```python
from build123d import *

# Parameters (mm, degrees)
BASPROSKE_W             = 12
BASPROSKE_H             = 25.5
TOOTHCUT_DEPTH          = 39.006578378
TEETHCUTS_COUNT         = 15
TEETHCUTS_ANGLE         = 336
BORSKE_R                = 10
BORE_DEPTH              = 50.0000508
CUT_EXTRUDE1_DEPTH      = 38.954121274
CUT_EXTRUDE1_DEPTH_BACK = 38.954121274
SKETCH1_W               = 6
SKETCH1_H               = 6


with BuildPart() as part:
    # BasProSke → Base-Revolve (revolve)
    with BuildSketch(Plane(origin=(0, 0, 0), x_dir=(1, 0, 0), z_dir=(0, 1, 0)), mode=Mode.PRIVATE) as base_revolve_sk:
        with Locations((6, 12.75)):
            Rectangle(BASPROSKE_W, BASPROSKE_H)
    revolve(base_revolve_sk.sketch.rotate(Axis((-10, 0, 0), (1, 0, 0)), 180), axis=Axis((-10, 0, 0), (1, 0, 0)))

    # TooCutSke → ToothCut (cut, through all)
    with BuildSketch(Plane(origin=(0, 0, 0), x_dir=(0, 0, -1), z_dir=(1, 0, 0))):
        with BuildLine():
            ThreePointArc((1.584594428, 18.681918036), (0, 18.749), (-1.584594428, 18.681918036))
            ThreePointArc((-1.584594428, 18.681918036), (-2.465052499, 22.206073835), (-4.666912141, 25.095138498))
            ThreePointArc((-4.666912141, 25.095138498), (0, 25.5254), (4.666912141, 25.095138498))
            ThreePointArc((4.666912141, 25.095138498), (2.465052499, 22.206073835), (1.584594428, 18.681918036))
        make_face()
    toothcut = extrude(amount=TOOTHCUT_DEPTH, mode=Mode.SUBTRACT)

    # TeethCuts: ToothCut ×15 about axis
    teethcuts_axis = Axis((-10, 0, 0), (1, 0, 0))
    for i in range(1, TEETHCUTS_COUNT):
        add(toothcut.rotate(teethcuts_axis, i * TEETHCUTS_ANGLE / (TEETHCUTS_COUNT - 1)), mode=Mode.SUBTRACT)

    # BorSke → Bore (cut, symmetric)
    with BuildSketch(Plane(origin=(0, 0, 0), x_dir=(0, 0, -1), z_dir=(1, 0, 0))):
        with Locations(Location((0, 0, 0), (0, 0, 180))):
            Circle(BORSKE_R)
    extrude(amount=BORE_DEPTH, both=True, mode=Mode.SUBTRACT)

    # Sketch1 → Cut-Extrude1 (cut, two sides: drawn at the far end of the back side and taken through both)
    with BuildSketch(Plane(origin=(0, 0, 0), x_dir=(0, 0, -1), z_dir=(1, 0, 0)).offset(-CUT_EXTRUDE1_DEPTH_BACK)):
        with Locations((0, 10)):
            Rectangle(SKETCH1_W, SKETCH1_H)
    extrude(amount=CUT_EXTRUDE1_DEPTH + CUT_EXTRUDE1_DEPTH_BACK, mode=Mode.SUBTRACT)


solid = part.part
```
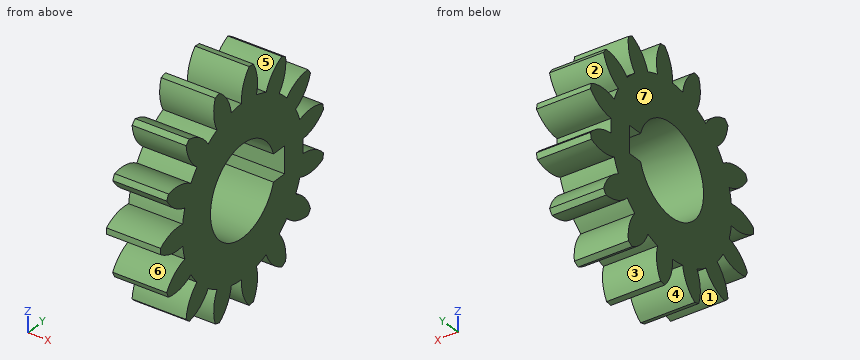
Work out the finished part from the listing and answer in its coordinate system (mm). Face numbers are marked on the shaded views. A direction names the side the tool comes from. Coordinates: 2 decimals unless noted, no trailing zeros. Loops run counter-clockwise (first coordinate to the right, second up) from the corner with the lowest first, then second, coordinate; pieces in that order, holes last. Notation, with made-up numbers: (-5.75, 62.5) -> (21.25, 62.5) arc R26 cw to (21.25, 82.5) -> close; hole circle Ø1 at (-3, 1). An arc over 180 degrees is marked (long way). Answer as CSV lines item,"result".
Q1. A tool of negligible diameter and unlimited length cuts with its end or side. For the marked faces 1, 2 and 3, from which of +Z, -Z, +X, -X, +Y, -Y can it reach the whole face along a straight path? Write none if from no direction.
Findings:
face 1,"-Z, +X, -X"
face 2,"+X, -X, +Y"
face 3,"+X, -X"
Q2. The part is cut by section B-B on y = -5.5. Write down the section's boundary in (x, z), and give its area (3 significant figures).
Findings:
outline,"(0, -22.84) -> (12, -22.84) -> (12, -8.35) -> (0, -8.35) -> close; (0, 8.35) -> (12, 8.35) -> (12, 22.84) -> (0, 22.84) -> close"
area,"348 mm²"
Q3. Each of these flat-tipped pins is pushed along its axis until it touches: pin 1 (1.7 mm diameter, centred on x = 4.5, y = 11.5, fed in from +Z); pin 2 (1.5 mm diameter, centred on x = 8, z = 10, fed in from -Y); pin 3 (1.5 mm diameter, centred on x = 9, y = -17.5, fed in from +Z). Where does it stop, or does it pass through?
Findings:
pin 1,"stops at z = 22.41"
pin 2,"stops at y = -23.56"
pin 3,"stops at z = 19.23"
Q4. For a pull along Y with two mould halves and no side action, classify the marked faces 4, 5, 6 and 7 as +Y half, -Y half, draft (parallel to the pull), parting line (faces both ways), or undercut.
Findings:
face 4,"undercut"
face 5,"undercut"
face 6,"-Y half"
face 7,"draft"
Q5. The part is cut by section A-A on z = 0. Write down the section's boundary in (x, y), and give its area (3 significant figures).
Findings:
outline,"(0, -25.5) -> (12, -25.5) -> (12, -10) -> (0, -10) -> close; (0, 13) -> (12, 13) -> (12, 18.75) -> (0, 18.75) -> close"
area,"255 mm²"
Q6. Find the intervals of material crossed by probe 1 along Y at (x, z) = (5.5, -22); probe 2 along Y at (x, z) = (4.75, -1.5); probe 3 along Z at (x, y) = (10.75, 7), in increasing order.
Findings:
probe 1,"y = -8.95 to -4.88, 0.02 to 4.5, 11.33 to 12.89"
probe 2,"y = -24.15 to -9.89, 13 to 18.69"
probe 3,"z = -17.39 to -7.14, 7.14 to 17.39"
